Autodesk Inventor part; units mm, degrees
ref_plane "YZ Plane" through (0, 0, 0) normal (1, 0, 0) x (0, 1, 0)
ref_plane "XZ Plane" through (0, 0, 0) normal (0, 1, 0) x (-1, 0, 0)
ref_plane "XY Plane" through (0, 0, 0) normal (0, 0, 1) x (1, 0, 0)
sketch "スケッチ1" plane through (0, 0, 0) normal (0, 0, 1) x (1, 0, 0)
  line L0 (0, 0) -> (40, 0)
  line L1 (40, 0) -> (40, 19.3)
  line L2 (40, 19.3) -> (20, 19.3)
  line L3 (20, 19.3) -> (20, 25.3)
  line L4 (20, 25.3) -> (0, 25.3)
  line L5 (0, 25.3) -> (0, 0)
  line L6 (20, 24.8) -> (19.5, 25.3)
  line L7 (10, 25.3) -> (10, 21.3)
  line L8 (10, 21.3) -> (0, 21.3)
  line L9 (10.5, 25.3) -> (10, 24.8)
  dimension "d0" = 40
  dimension "d1" = 19.3
  dimension "d2" = 20
  dimension "d3" = 6
  dimension "d4" = 135
  dimension "d5" = 0.5
  dimension "d6" = 4
  dimension "d7" = 0.5
  dimension "d8" = 45
revolve "回転1" add sketch "スケッチ1" angle 360 about axis through (0, 25.3, 0) along (0, -1, 0) contours L5 L8 L7 L9 L4 L6 L3 L2 L1 L0
sketch "スケッチ2" plane through (0, 19.3, 0) normal (0, 1, 0) x (1, 0, 0)
  point P0 (0, 0)
  point P1 (0, -35)
  point P2 (0, 0)
  point P3 (35, 0)
  point P4 (0, 35)
  point P5 (-35, 0)
  dimension "d12" = 360
hole "穴1" at (0, 19.3, 35) at (0, 19.3, 0) at (35, 19.3, 0) at (0, 19.3, -35) at (-35, 19.3, 0) direction (0, -1, 0) diameter 2.459 depth 6 tip angle 118
sketch "スケッチ3" plane through (0, 25.3, 0) normal (0, 1, 0) x (1, 0, 0)
  point P0 (0, 0)
  point P1 (0, 15.75)
  point P2 (-15.75, 0)
  point P3 (0, -15.75)
  point P4 (15.75, 0)
  dimension "d21" = 15.75
  dimension "d24" = 360
hole "穴2" at (0, 25.3, -15.75) at (-15.75, 25.3, 0) at (0, 25.3, 15.75) at (15.75, 25.3, 0) direction (0, -1, 0) diameter 4.4587 depth 8 tip angle 118
sketch "スケッチ4" plane through (0, 25.3, 0) normal (0, 1, 0) x (1, 0, 0)
  circle A0 centre (0, 0) radius 1.2295
  circle A1 centre (0, 0) radius 15.75 construction
  line L0 (-11.1369, 11.1369) -> (0, 0) construction
  line L1 (0, 0) -> (-15.75, 0) construction
  dimension "d33" = 31.5
  dimension "d34" = 45
hole "穴3" at (-11.1369, 25.3, -11.1369) direction (0, -1, 0) diameter 5 depth 8 tip angle 118
properties part number "マニピュレータ手首ISO9409"
Could you check a few things on this model? Use its own coordinates, in mm. A direction names the side the tool comes from. Give positions to 0.01 mm unless a question says otherwise; leave off trailing zeros. Order: outer loops, then holes, each group sorted by start corner. A loop starts at its lowest first (then second) coordinate and runs counter-clockwise, first axis right, second up.
1. I need wall thicknesses on L1, parallel to Z at x = 0, y = 17.35; L2, parallel to Y at x = 8.5, z = 24.5; L3, parallel to X at y = 21.5, z = -4.5. Which ranges of each line are inside material? Lowest first, please.
2. For faces 1 (the flat face through (8, 25.3, -8)), 2 (the cylindrical face through (0.748, 16.258, -0.976)), 3 (the cylindrical face through (-36.22, 16.26, -0.16)), which set-ups out of +Z, -Z, +X, -X, +Y, -Y let a thin tool reach every point of the face, with its end or its side?
3. We'd pull the mould along Y, two halves only. Please class faces 4 (the cylindrical face through (-4.336, 22.088, 19.524)), 5 (the flat face through (-1, 0, 1)), 6 (the conical face through (-0.21, 12.69, -0.05)): pulls with the +Y half, pulls with the -Y half, needs draft (parallel to the pull), parting line crosses it, or undercut.
4. Will these pins go through, and if not, where does the flat tip stop? P1, Ø8, axis at y = 13, z = -24, coming from the -X side; P2, Ø8, axis at x = 17.5, y = 9.5, coming from the +Z side; P3, Ø16, axis at x = 0, z = 0, coming from the +Y side.
5. Suppose I cut it at C-C (x = 22). List the corners of the cut face in (y, z) for me.
6. Suppose I cut it at A-A (z = -24). List the corners of the cut face in (x, y) for me.
7. Suppose I cut it at B-B (y = 1.5). List the corners of the cut face in (x, z) for me, plus the area to 3 significant figures.
Solved:
1. L1: z = -40 to -36.23, -33.77 to -17.98, -13.52 to -1.23, 1.23 to 13.52, 17.98 to 33.77, 36.23 to 40
1. L2: y = 0 to 19.3
1. L3: x = -19.49 to -8.93, 8.93 to 19.49
2. face 1: +Z, -Z, +X, -X, +Y
2. face 2: none
2. face 3: +Y
3. face 4: needs draft
3. face 5: pulls with the -Y half
3. face 6: undercut
4. P1: stops at x = -34.64
4. P2: stops at z = 37.65
4. P3: stops at y = 21.3
5. outline: (0, -33.41) - (19.3, -33.41) - (19.3, 33.41) - (0, 33.41) - close
6. outline: (-32, 0) - (32, 0) - (32, 19.3) - (-32, 19.3) - close
7. outline: circle Ø80 at (0, 0)
7. area: 5,030 mm2
